Build history of the part. All positions in model axes, mm. Face numbers are marked on the shaded views. A direction names the side the tool comes from. Give positions to 0.01 mm unless a question says otherwise; leave off trailing zeros. Loops run counter-clockwise (first coordinate to the right, second up) from the corner with the lowest first, then second, coordinate; pieces in that order, holes last.
1) Two-plate mould, pull along Y, no slides. Class the marked faces 1, 2, 3 and 4: +Y half, -Y half, draft (parallel to the pull), parting line (faces both ways), or undercut.
2) Flat gauge pins, fed straight in: P1, Ø1.7, axis at x = -6, y = -11.5, coming from the -Z side; P2, Ø1.2, axis at x = -6, y = -0.5, coming from the -Z side; P3, Ø2, axis at x = -6, z = -6, coming from the -Y side. Where does each tip first touch, or does it go through?
3) Band-saw the part on D-D on y = -13.5. List the corners of the cut face in (x, z), then the cut area to 3 significant figures.
4) Band-saw the part on A-A on x = -5.5. List the corners of the cut face in (y, z).
5) 3-axis set-ups, long thin cutter, end or side, ignore diameter. For the marked faces 5, 6 and 7: which of +Z, -Z, +X, -X, +Y, -Y reach the whole face in a straight line?
6) Band-saw the part on C-C on z = -6.45. List the corners of the cut face in (x, y).
7) Band-saw the part on B-B on y = 0. List the corners of the cut face in (x, z), then the cut area to 3 significant figures.
8) Wall check: line 1 (Y direction, x = -5.5, z = -3.05); line 2 (Y direction, x = -6.5, z = -3.35); line 3 (Y direction, x = -5.5, z = -5.25). Give the ranges that are in metal, low to high.
```python
from build123d import *

# Parameters (mm, degrees)
SKETCH1_R           = 3.5687
SKETCH1_R_2         = 2
BOSS_EXTRUDE1_DEPTH = 4.191
SKETCH5_R           = 2
SKETCH5_R_2         = 1.143
BOSS_EXTRUDE2_DEPTH = 0.2226
BOSS_EXTRUDE3_START = -1.524
SKETCH6_R           = 1.25
BOSS_EXTRUDE3_DEPTH = 1.524


with BuildPart() as part:
    # Sketch1 → Boss-Extrude1 (new body)
    with BuildSketch(Plane.XY.offset(-7.032965862)):
        with Locations((-5.5, 0)):
            Circle(SKETCH1_R)
        with Locations((-5.5, 0)):
            Circle(SKETCH1_R_2, mode=Mode.SUBTRACT)
    extrude(amount=BOSS_EXTRUDE1_DEPTH)

    # Sketch5 → Boss-Extrude2 (add)
    with BuildSketch(Plane.XY.offset(-4.232965862)):
        with Locations((-5.5, 0)):
            Circle(SKETCH5_R)
        with Locations((-5.5, 0)):
            Circle(SKETCH5_R_2, mode=Mode.SUBTRACT)
    extrude(amount=BOSS_EXTRUDE2_DEPTH)

    # Sketch6 → Boss-Extrude3 (add)
    with BuildSketch(Plane.XY.offset(-2.841965862).offset(BOSS_EXTRUDE3_START)):
        with BuildLine():
            Line((-3.75375, -14.09065), (-2.68695, -2.195989387))
            ThreePointArc((-2.68695, -2.195989387), (-5.5, -3.5687), (-8.31305, -2.195989387))
            Line((-8.31305, -2.195989387), (-7.24625, -14.09065))
            ThreePointArc((-7.24625, -14.09065), (-5.5, -15.8369), (-3.75375, -14.09065))
        make_face()
        with Locations((-5.5, -12.84065)):
            Circle(SKETCH6_R, mode=Mode.SUBTRACT)
    extrude(amount=BOSS_EXTRUDE3_DEPTH)


solid = part.part
```
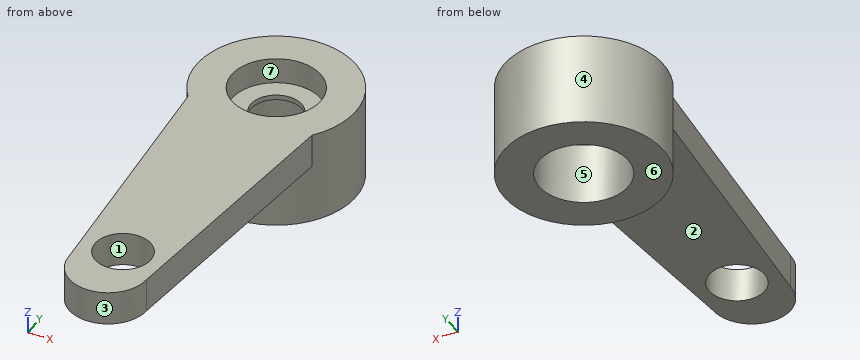
Findings below:
1. face 1: undercut
1. face 2: draft
1. face 3: -Y half
1. face 4: parting line
2. P1: stops at z = -4.37
2. P2: stops at z = -4.23
2. P3: stops at y = -3.57
3. outline: (-7.3, -4.37) - (-6.56, -4.37) - (-6.56, -2.84) - (-7.3, -2.84) - close; (-4.44, -4.37) - (-3.7, -4.37) - (-3.7, -2.84) - (-4.44, -2.84) - close
3. area: 2.25 mm2
4. outline: (-15.84, -4.37) - (-14.09, -4.37) - (-14.09, -2.84) - (-15.84, -2.84) - close; (-11.59, -4.37) - (-3.57, -4.37) - (-3.57, -7.03) - (-2, -7.03) - (-2, -4.23) - (-1.14, -4.23) - (-1.14, -4.01) - (-2, -4.01) - (-2, -2.84) - (-11.59, -2.84) - close; (1.14, -4.23) - (2, -4.23) - (2, -7.03) - (3.57, -7.03) - (3.57, -2.84) - (2, -2.84) - (2, -4.01) - (1.14, -4.01) - close
5. face 5: -Z
5. face 6: -Z, +X, -X, +Y, -Y
5. face 7: +Z
6. outline: circle Ø7.14 at (-5.5, 0); hole circle Ø4 at (-5.5, 0)
7. outline: (-9.07, -7.03) - (-7.5, -7.03) - (-7.5, -4.23) - (-6.64, -4.23) - (-6.64, -4.01) - (-7.5, -4.01) - (-7.5, -2.84) - (-9.07, -2.84) - close; (-4.36, -4.23) - (-3.5, -4.23) - (-3.5, -7.03) - (-1.93, -7.03) - (-1.93, -2.84) - (-3.5, -2.84) - (-3.5, -4.01) - (-4.36, -4.01) - close
7. area: 13.5 mm2
8. line 1: y = -15.84 to -14.09, -11.59 to -2, 2 to 3.57
8. line 2: y = -15.52 to -13.59, -12.09 to -1.73, 1.73 to 3.43
8. line 3: y = -3.57 to -2, 2 to 3.57
